The drawing under review shows one solid part. Ordinate dimensions are in mm from its lowest x, y, z. Round coordinates to 2 decimals unless told otherwise and drop trailing zeros. Order: outer loops, then holes, each group sorted by start corner. A loop starts at its lowest first (then second) coordinate and runs counter-clockwise, first axis right, second up. Notation, with made-up numbers: (-29.75, 11.5) -> (-12.75, 11.5) arc R16 ccw to (-12.75, 20.5) -> close; hole circle Ø3 at (60, 38.5). An arc over 180 degrees is marked (long way). Put each result on its own line as item: value. Start each with the question number.
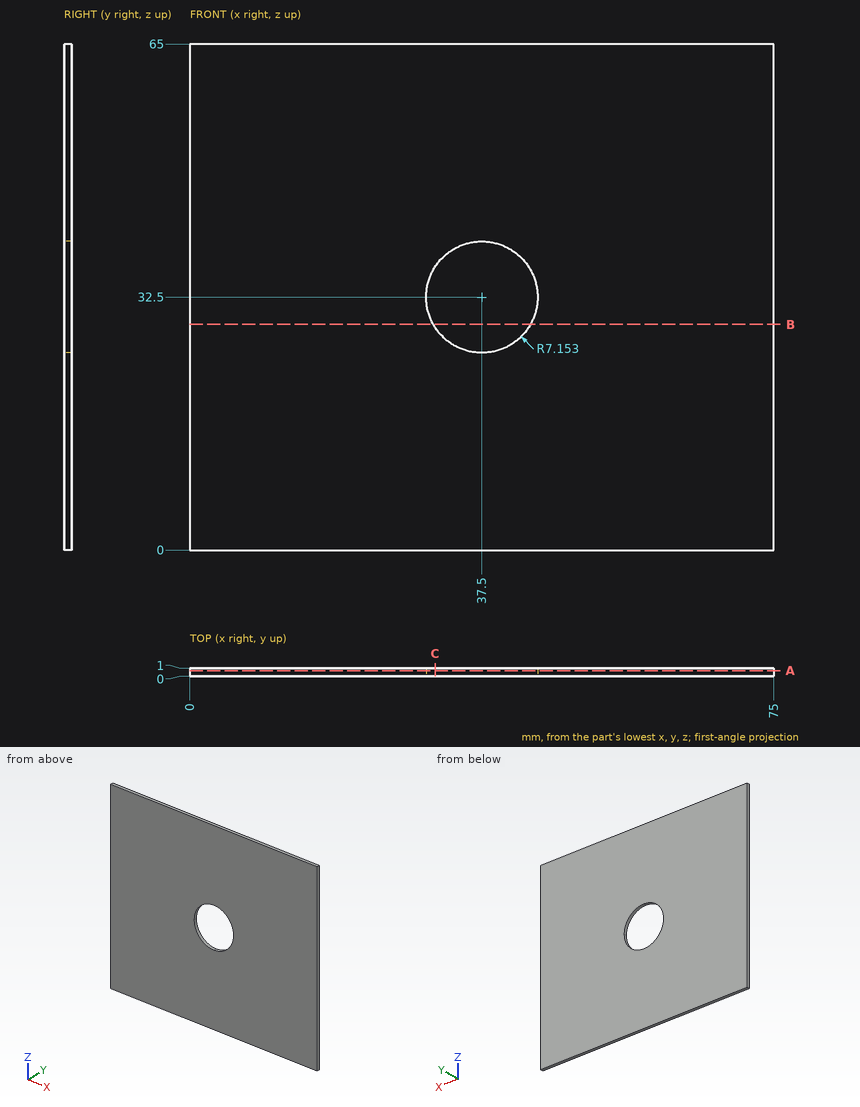
Item 1: Consider section B-B, the plane z = 29. Write out the cut boundary in (x, y).
Item 2: Consider section A-A, the plane y = 0.7. Write out the cut boundary in (x, z) (1 decimal), plus the area to 3 significant figures.
Item 3: For L1, parallel to Z at x = 38, y = 0.4 (1 decimal); L2, parallel to Z at x = 34, y = 0.1; L3, parallel to X at y = 0.5, z = 37.5 (1 decimal), list the stretches that pass through material, from the lowest coordinate up.
Item 4: Consider section C-C, the plane x = 31.5. Write out the cut boundary in (y, z).
Evaluation:
1. outline: (0, 0) -> (31.26, 0) -> (31.26, 1) -> (0, 1) -> close; (43.74, 0) -> (75, 0) -> (75, 1) -> (43.74, 1) -> close
2. outline: (0, 0) -> (75, 0) -> (75, 65) -> (0, 65) -> close; hole (30.3, 32.5) arc R7.2 ccw to (37.5, 25.3) arc R7.2 ccw to (44.7, 32.5) arc R7.2 ccw to (37.5, 39.7) arc R7.2 ccw to start
2. area: 4,710 mm^2
3. L1: z = 0 to 25.4, 39.6 to 65
3. L2: z = 0 to 26.26, 38.74 to 65
3. L3: x = 0 to 32.4, 42.6 to 75
4. outline: (0, 0) -> (1, 0) -> (1, 28.61) -> (0, 28.61) -> close; (0, 36.39) -> (1, 36.39) -> (1, 65) -> (0, 65) -> close
